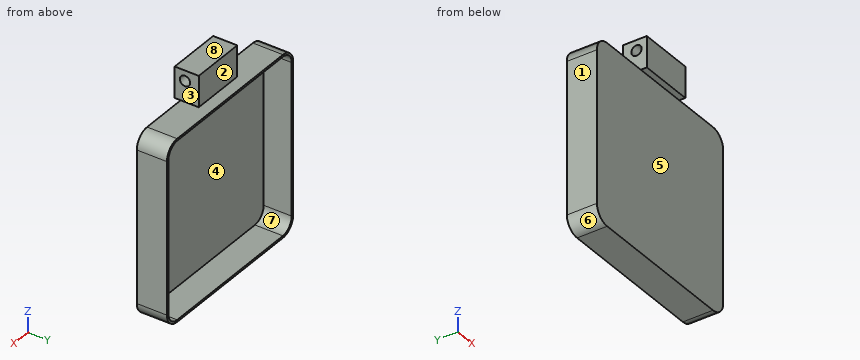
Autodesk Inventor part; units mm, degrees
ref_plane "YZ Plane" through (0, 0, 0) normal (1, 0, 0) x (0, 1, 0)
ref_plane "XZ Plane" through (0, 0, 0) normal (0, 1, 0) x (-1, 0, 0)
ref_plane "XY Plane" through (0, 0, 0) normal (0, 0, 1) x (1, 0, 0)
sketch "Szkic1" plane through (0, 0, 0) normal (0, 1, 0) x (-1, 0, 0)
  line L0 (52.5, 52.5) -> (-52.5, 52.5)
  line L1 (-52.5, 52.5) -> (-52.5, -52.5)
  line L2 (-52.5, -52.5) -> (52.5, -52.5)
  line L3 (52.5, -52.5) -> (52.5, 52.5)
  point P0 (0, 0)
  dimension "d0" = 105
  dimension "d1" = 105
  dimension "d2" = 52.5
  dimension "d3" = 52.5
extrude "Wyciągnięcie proste1" add sketch "Szkic1" along normal blind 17.5
fillet "Zaokrąglenie1" radius 8.5 4 edges at (52.5, 8.75, 52.5) (-52.5, 8.75, 52.5) (52.5, 8.75, -52.5) (-52.5, 8.75, -52.5)
shell "Skorupa1" thickness 1.2 removed faces 1 at (-20.3333, 17.5, -17.5)
sketch "Szkic4" plane through (-44, 0, 52.5) normal (0, 0, 1) x (1, 0, 0)
  line L0 (0, 0) -> (88, 0)
  line L1 (28, -3.5) -> (60, -3.5)
  line L2 (60, -3.5) -> (60, 10.5)
  line L3 (60, 10.5) -> (28, 10.5)
  line L4 (28, 10.5) -> (28, -3.5)
  line L5 (0, 17.5) -> (88, 17.5)
  point P0 (60, 0)
  point P1 (44, 0)
  point P2 (44, 17.5)
  dimension "d21" = 32
  dimension "d22" = 16
  dimension "d23" = 21
  dimension "d24" = 14
extrude "Wyciągnięcie proste4" add sketch "Szkic4" along normal blind 18
sketch "Szkic6" plane through (-16, -3.5, 52.5) normal (-1, 0, 0) x (0, 0, 1)
  circle A0 centre (12, 6) radius 3
  line L0 (0, 3.5) -> (0, 21)
  line L1 (0, 0) -> (18, 0)
  point P0 (-52.5, 3.5)
  dimension "d29" = 6
  dimension "d30" = 12
  dimension "d31" = 3
extrude "Wyciągnięcie proste6" cut sketch "Szkic6" against normal blind 50
properties part number "lampa"
The model under review builds one solid part; all positions refer to its coordinate system, in mm. Face numbers are marked on the shaded views. A direction names the side the tool comes from. Round coordinates to 2 decimals unless told otherwise and drop trailing zeros. Loops run counter-clockwise (first coordinate to the right, second up) from the corner with the lowest first, then second, coordinate; pieces in that order, holes last.
1) Consider section D-D on z = 0. State the section outline as (x, y) points, then the cut area to 3 significant figures.
Values follow:
outline: (-52.5, 0) - (52.5, 0) - (52.5, 17.5) - (51.3, 17.5) - (51.3, 1.2) - (-51.3, 1.2) - (-51.3, 17.5) - (-52.5, 17.5) - close
area: 165 mm2
2) Consider section B-B on y = 12.5. State the section outline as (x, z) points, then the cut area to 3 significant figures.
Values follow:
outline: (-52.5, -44) arc R8.5 ccw to (-44, -52.5) - (44, -52.5) arc R8.5 ccw to (52.5, -44) - (52.5, 44) arc R8.5 ccw to (44, 52.5) - (-44, 52.5) arc R8.5 ccw to (-52.5, 44) - close; hole (-51.3, -44) arc R7.3 ccw to (-44, -51.3) - (44, -51.3) arc R7.3 ccw to (51.3, -44) - (51.3, 44) arc R7.3 ccw to (44, 51.3) - (-44, 51.3) arc R7.3 ccw to (-51.3, 44) - close
area: 482 mm2
3) The part is to be moulded in two halves that separate along X. For the marked faces 6, 7 and 8, say which applies: pulls with the +X half, pulls with the -X half, needs draft (parallel to the pull), parting line crosses it, or undercut.
Values follow:
face 6: pulls with the -X half
face 7: undercut
face 8: needs draft
4) Wall thickness on line 1 along X through (y, z) = (15.5, -1); line 2 along Y through (x, z) = (8.5, 64.5): over which ranges is each line inside the solid? List them lowest first.
Values follow:
line 1: x = -52.5 to -51.3, 51.3 to 52.5
line 2: y = -3.5 to -0.5, 5.5 to 10.5
5) Clearance check with flat-ended pins moving along their axes: P1, Ø20, axis at x = -0.5, z = 57.5, coming from the +Y side; P2, Ø3, axis at x = 2.5, y = -2, coming from the -Z side; P3, Ø8, axis at x = -31.5, z = -9.5, coming from the -Y side; P4, Ø8, axis at y = 2.5, z = 64.5, coming from the +X side. State where each tip first meets the part, or that it passes through.
Values follow:
P1: stops at y = 17.5
P2: stops at z = 52.5
P3: stops at y = 0
P4: stops at x = 16
6) Consider section C-C on x = 1.5. State the section outline as (y, z) points.
Values follow:
outline: (-3.5, 52.5) - (0, 52.5) - (0, -52.5) - (17.5, -52.5) - (17.5, -51.3) - (1.2, -51.3) - (1.2, 51.3) - (17.5, 51.3) - (17.5, 52.5) - (10.5, 52.5) - (10.5, 70.5) - (-3.5, 70.5) - close; hole circle Ø6 at (2.5, 64.5)
7) Tool access review of the marked faces 1, 2, 3, 4 and 5: name each direction out of +Z, -Z, +X, -X, +Y, -Y from which nothing blocks a thin tool from reaching the whole face with its end or side.
Values follow:
face 1: +Z, -Z, -X, +Y, -Y
face 2: +Z, +X, -X, +Y
face 3: +Z, +X, +Y, -Y
face 4: +Y
face 5: -Z, +X, -X, -Y
8) Consider section A-A on z = 64.5. State the section outline as (x, y) points.
Values follow:
outline: (-16, -3.5) - (16, -3.5) - (16, -0.5) - (-16, -0.5) - close; (-16, 5.5) - (16, 5.5) - (16, 10.5) - (-16, 10.5) - close
